Autodesk Inventor part; units mm, degrees
ref_plane "YZ Plane" through (0, 0, 0) normal (1, 0, 0) x (0, 1, 0)
ref_plane "XZ Plane" through (0, 0, 0) normal (0, 1, 0) x (-1, 0, 0)
ref_plane "XY Plane" through (0, 0, 0) normal (0, 0, 1) x (1, 0, 0)
sketch "Sketch1" plane through (0, 0, 0) normal (0, 0, 1) x (1, 0, 0)
  circle A0 centre (0, 0) radius 3.85
  dimension "d0" = 7.7
extrude "Extrusion1" add sketch "Sketch1" along normal blind 10.2
sketch "Sketch2" plane through (0, 0, 10.2) normal (0, 0, 1) x (1, 0, 0)
  circle A0 centre (0, 0) radius 4
  dimension "d3" = 8
extrude "Extrusion2" add sketch "Sketch2" along normal blind 2 draft 75
sketch "Sketch3" plane through (0, 0, 12.2) normal (0, 0, 1) x (1, 0, 0)
  circle A0 centre (0, 0) radius 15
  dimension "d6" = 30
extrude "Extrusion3" add sketch "Sketch3" along normal blind 10
sketch "Sketch5" plane through (0, 0, 22.2) normal (0, 0, 1) x (1, 0, 0)
  circle A0 centre (0, 0) radius 11.25
  dimension "d11" = 22.5
extrude "Extrusion5" cut sketch "Sketch5" against normal blind 7
sketch "Sketch6" plane through (0, 0, 0) normal (0, 0, -1) x (-1, 0, 0)
  circle A0 centre (0, 0) radius 2.55
  dimension "d14" = 5.1
extrude "Extrusion6" cut sketch "Sketch6" against normal blind 1.8
sketch "Sketch7" plane through (0, 0, 1.8) normal (0, 0, -1) x (-1, 0, 0)
  point P0 (0, 0)
sketch "Sketch8" plane through (0, 0, 1.8) normal (0, 0, -1) x (-1, 0, 0)
  line L0 (-1.55, 2.0667) -> (1.55, 2.0667)
  line L1 (1.55, 2.0667) -> (1.55, -2.0667)
  line L2 (1.55, -2.0667) -> (-1.55, -2.0667)
  line L3 (-1.55, -2.0667) -> (-1.55, 2.0667)
  line L4 (-1.55, 2.0667) -> (1.55, -2.0667) construction
  line L5 (1.55, 2.0667) -> (-1.55, -2.0667) construction
  circle A0 centre (0, 0) radius 2.5833
  arc A1 (1.55, 2.0667) -> (-1.55, 2.0667) centre (0, 0) ccw
  arc A2 (-1.55, -2.0667) -> (1.55, -2.0667) centre (0, 0) ccw
  arc A3 (1.55, 2.0667) -> (-1.55, 2.0667) centre (0, 0.6019) ccw
  arc A4 (-1.55, -2.0667) -> (1.55, -2.0667) centre (0, -0.6159) ccw
  dimension "d17" = 3.1
extrude "Extrusion7" cut sketch "Sketch8" against normal blind 8 contours A0 L0 | L0 L1 L2 L3 | L2 A0
sketch "Sketch9" plane through (0, 0, 12.2) normal (0, 0, -1) x (-1, 0, 0)
  line L0 (-5, -12) -> (5, -12)
  line L1 (5, -12) -> (5, -35)
  line L2 (5, -35) -> (-5, -35)
  line L3 (-5, -35) -> (-5, -12)
  circle A0 centre (0, 0) radius 15
  point P0 (0, -15)
  dimension "d25" = 20
  dimension "d30" = 5
  dimension "d31" = 5
  dimension "d32" = 3
extrude "Extrusion8" add sketch "Sketch9" against normal blind 10 contours L0 L1 A0 L3 | A0 L1 L2 L3 picked at (0.5652, -12.968)
sketch "Sketch10" plane through (0, 0, 12.2) normal (0, 0, -1) x (-1, 0, 0)
  circle A0 centre (0, -31) radius 2.25
  line L0 (-5, -35) -> (5, -35)
  point P0 (0, 0)
  dimension "d33" = 4.5
  dimension "d34" = 4
extrude "Extrusion9" cut sketch "Sketch10" against normal through all
sketch "Sketch11" plane through (0, 0, 22.2) normal (0, 0, 1) x (1, 0, 0)
  point P0 (0, 0)
sketch "Sketch12" plane through (0, 0, 0) normal (0, 0, -1) x (-1, 0, 0)
  line L0 (0, 4.2717) -> (0.5, 4.2717)
  line L1 (0.5, 4.2717) -> (0.5, 22.715)
  line L2 (0.5, 22.715) -> (-0.5, 22.715)
  line L3 (-0.5, 22.715) -> (-0.5, 4.2717)
  line L4 (-0.5, 4.2717) -> (0, 4.2717)
  point P0 (0, 0)
  dimension "d37" = 0.5
  dimension "d38" = 1
extrude "Extrusion10" cut sketch "Sketch12" against normal through all
properties part number "Motorshaft"
Part model, mm, in its own coordinate system. A direction names the side the tool comes from. Give positions to 0.01 mm unless a question says otherwise; leave off trailing zeros. Order: outer loops, then holes, each group sorted by start corner. A loop starts at its lowest first (then second) coordinate and runs counter-clockwise, first axis right, second up. Notation, with made-up numbers: (87.5, 66.5) - (104.5, 66.5) arc R17 ccw to (104.5, 71.5) - close; hole circle Ø10 at (75, 10.25). An arc over 180 degrees is marked (long way). Use a Markdown table: item, result.
1) Saw through at C-C on z = 13.5. List the corners of the cut face in (x, y).
Checked values:
| item | result |
|---|---|
| outline | (-5, -35) - (5, -35) - (5, -14.14) arc R15 ccw to (0.5, 14.99) - (0.5, 4.27) - (-0.5, 4.27) - (-0.5, 14.99) arc R15 ccw to (-5, -14.14) - close; hole circle Ø4.5 at (0, -31) |
2) Probe L1, parallel to X at y = 0, z = 18.5; L2, parallel to Y at x = 0, z = 1.2; L3, parallel to Y at x = 0, z = 18. List the from-to ranges inside material, lowest first. Write a range as from..to.
Checked values:
| item | result |
|---|---|
| L1 | -15..-11.25, 11.25..15 |
| L2 | -3.85..-2.55, 2.55..3.85 |
| L3 | -35..-33.25, -28.75..-11.25 |
3) Saw through at B-B on y = -31. List the corners of the cut face in (x, z).
Checked values:
| item | result |
|---|---|
| outline | (-5, 12.2) - (-2.25, 12.2) - (-2.25, 22.2) - (-5, 22.2) - close; (2.25, 12.2) - (5, 12.2) - (5, 22.2) - (2.25, 22.2) - close |
4) Two-plate mould, pull along X, no slides. Class faces 3 (the flat face through (0, -14, 12.2)), 4 (the flat face through (5, -25, 17)), 5 (the cylindrical face through (-1.18, -2.26, 0.89)): +X half, -X half, draft (parallel to the pull), parting line (faces both ways), or undercut.
Checked values:
| item | result |
|---|---|
| face 3 | draft |
| face 4 | +X half |
| face 5 | undercut |
5) Saw through at D-D on z = 17.25. List the corners of the cut face in (x, y), plus the area to 3 significant figures.
Checked values:
| item | result |
|---|---|
| outline | (-5, -35) - (5, -35) - (5, -14.14) arc R15 ccw to (0.5, 14.99) - (0.5, 11.24) arc R11.25 cw (long way) to (-0.5, 11.24) - (-0.5, 14.99) arc R15 ccw to (-5, -14.14) - close; hole circle Ø4.5 at (0, -31) |
| area | 492 mm² |
6) 3-axis set-ups, long thin cutter, end or side, ignore diameter. For faces 1 (the flat face through (0, 4.272, 13)), 2 (the flat face through (0, 0, 15.2)): which of +Z, -Z, +X, -X, +Y, -Y reach the whole face in a straight line?
Checked values:
| item | result |
|---|---|
| face 1 | +Z, -Z, +Y |
| face 2 | +Z |
7) Flat gauge pins, fed straight in: P1, Ø2, axis at y = -0.5, z = 5, coming from the -X side; P2, Ø1, axis at x = 0.5, y = 8.5, coming from the -Z side; P3, Ø8, axis at y = -29.5, z = 14, coming from the +X side; P4, Ø6, axis at y = -22, z = 9, coming from the -X side. Where does each tip first touch, or does it go through?
Checked values:
| item | result |
|---|---|
| P1 | x = -3.85 |
| P2 | z = 11.28 |
| P3 | x = 5 |
| P4 | through |
